from build123d import *

# Parameters (mm, degrees)
F0_W      = 50
F0_H      = 17
F1_DEPTH  = 5
F5_DEPTH  = 8
F8_DEPTH  = 8
F9_R      = 3.25
F10_DEPTH = 25
F11_R     = 0.75


with BuildPart() as f1:
    # F0 (on Top) → F1 (new body)
    with BuildSketch(Plane.XY):
        Rectangle(F0_W, F0_H)
    extrude(amount=F1_DEPTH)

    # F4 (on line) → F5 (join)
    with BuildSketch(Plane.YZ.offset(-12.25)):
        with BuildLine():
            ThreePointArc((0, 5), (6.0104076401, 7.4895923599), (8.5, 13.5))
            ThreePointArc((8.5, 13.5), (0, 22), (-8.5, 13.5))
            ThreePointArc((-8.5, 13.5), (-6.0104076401, 7.4895923599), (0, 5))
        make_face()
        with BuildLine():
            Line((8.5, 5), (8.5, 13.5))
            ThreePointArc((8.5, 13.5), (6.0104076401, 7.4895923599), (0, 5))
            Line((0, 5), (8.5, 5))
        make_face()
        with BuildLine():
            ThreePointArc((0, 5), (-6.0104076401, 7.4895923599), (-8.5, 13.5))
            Line((-8.5, 13.5), (-8.5, 5))
            Line((-8.5, 5), (0, 5))
        make_face()
    extrude(amount=F5_DEPTH)

    # F7 (on line) → F8 (join)
    with BuildSketch(Plane.YZ.offset(4.25)):
        with BuildLine():
            ThreePointArc((0, 5), (6.0104076401, 7.4895923599), (8.5, 13.5))
            ThreePointArc((8.5, 13.5), (0, 22), (-8.5, 13.5))
            ThreePointArc((-8.5, 13.5), (-6.0104076401, 7.4895923599), (0, 5))
        make_face()
        with BuildLine():
            Line((8.5, 5), (8.5, 13.5))
            ThreePointArc((8.5, 13.5), (6.0104076401, 7.4895923599), (0, 5))
            Line((0, 5), (8.5, 5))
        make_face()
        with BuildLine():
            ThreePointArc((0, 5), (-6.0104076401, 7.4895923599), (-8.5, 13.5))
            Line((-8.5, 13.5), (-8.5, 5))
            Line((-8.5, 5), (0, 5))
        make_face()
    extrude(amount=F8_DEPTH)

    # F9 (on face) → F10 (cut)
    with BuildSketch(Plane.YZ.offset(12.25)):
        with Locations((0, 13.5)):
            Circle(F9_R)
    extrude(amount=-F10_DEPTH, mode=Mode.SUBTRACT)

    # F11
    f11_edges = [f1.edges().sort_by_distance(p)[0] for p in [
        (18.625, 8.5, 5),
        (0, 8.5, 5),
        (-18.625, 8.5, 5),
        (-18.625, -8.5, 5),
        (-25, 0, 5),
        (0, -8.5, 5),
        (18.625, -8.5, 5),
        (25, 0, 5),
    ]]
    fillet(f11_edges, radius=F11_R)


solid = f1.part
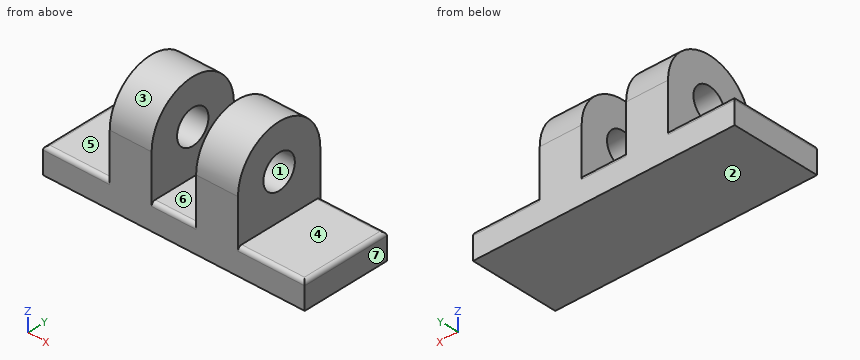
Geometry: final body of the model. Coordinates: model frame, mm. Face numbers are marked on the shaded views. A direction names the side the tool comes from. Round coordinates to 2 decimals unless told otherwise and drop trailing zeros. Loops run counter-clockwise (first coordinate to the right, second up) from the corner with the lowest first, then second, coordinate; pieces in that order, holes last.
Q1. Section C-C on x = 7. Return loops of the section in (y, z), plus the area to 3 significant figures.
Q2. Section B-B on z = 17.5. Return loops of the section in (x, y).
Q3. Section A-A on y = 0. Return loops of the section in (x, z), plus the area to 3 significant figures.
Q4. Section D-D on z = 14.75. Return loops of the section in (x, y).
Q5. Pin query (flat end, axial travel): P1, Ø6, axis at x = 21, y = -4, coming from the +Z side; P2, Ø6, axis at y = 0, z = 13.5, coming from the -X side; P3, Ø8.5, axis at y = 2.5, z = 17, coming from the -X side; P4, Ø6, axis at y = -6, z = 18.5, coming from the +X side. Return the tip coordinate at first contact, or that it passes through.
Q6. Material intervals for L1, parallel to X at y = -0.25, z = 19; L2, parallel to Z at x = -9, y = 0; L3, parallel to Y at x = 11, z = 13.25, sorted ascending.
Q7. Pull-direction query (Y, two-part tool) for the marked faces 1, 2 and 3; classes: released by +Y, released by -Y, zero draft, split by the parting line, or undercut.
Q8. Access query for the marked faces 4, 5, 6 and 7. Directions: +Z, -Z, +X, -X, +Y, -Y. A direction counts if a zero-diameter tool reaches every point of the face in a straight line with its end or side. Return the directions, or none.
Evaluation:
1. outline: (-8.5, 0) - (8.5, 0) - (8.5, 13.5) arc R8.5 ccw to (-8.5, 13.5) - close; hole circle Ø6.5 at (0, 13.5)
1. area: 310 mm2
2. outline: (-12.25, -7.5) - (-4.25, -7.5) - (-4.25, 7.5) - (-12.25, 7.5) - close; (4.25, -7.5) - (12.25, -7.5) - (12.25, 7.5) - (4.25, 7.5) - close
3. outline: (-25, 0) - (25, 0) - (25, 4.25) arc R0.75 ccw to (24.25, 5) - (12.25, 5) - (12.25, 10.25) - (4.25, 10.25) - (4.25, 5) - (-4.25, 5) - (-4.25, 10.25) - (-12.25, 10.25) - (-12.25, 5) - (-24.25, 5) arc R0.75 ccw to (-25, 4.25) - close; (-12.25, 16.75) - (-4.25, 16.75) - (-4.25, 22) - (-12.25, 22) - close; (4.25, 16.75) - (12.25, 16.75) - (12.25, 22) - (4.25, 22) - close
3. area: 418 mm2
4. outline: (-12.25, -8.41) - (-4.25, -8.41) - (-4.25, -3) - (-12.25, -3) - close; (-12.25, 3) - (-4.25, 3) - (-4.25, 8.41) - (-12.25, 8.41) - close; (4.25, -8.41) - (12.25, -8.41) - (12.25, -3) - (4.25, -3) - close; (4.25, 3) - (12.25, 3) - (12.25, 8.41) - (4.25, 8.41) - close
5. P1: stops at z = 5
5. P2: passes through
5. P3: stops at x = -12.25
5. P4: stops at x = 12.25
6. L1: x = -12.25 to -4.25, 4.25 to 12.25
6. L2: z = 0 to 10.25, 16.75 to 22
6. L3: y = -8.5 to -3.24, 3.24 to 8.5
7. face 1: undercut
7. face 2: zero draft
7. face 3: split by the parting line
8. face 4: +Z, +X, +Y, -Y
8. face 5: +Z, -X, +Y, -Y
8. face 6: +Z, +Y, -Y
8. face 7: +Z, -Z, +X, +Y, -Y
